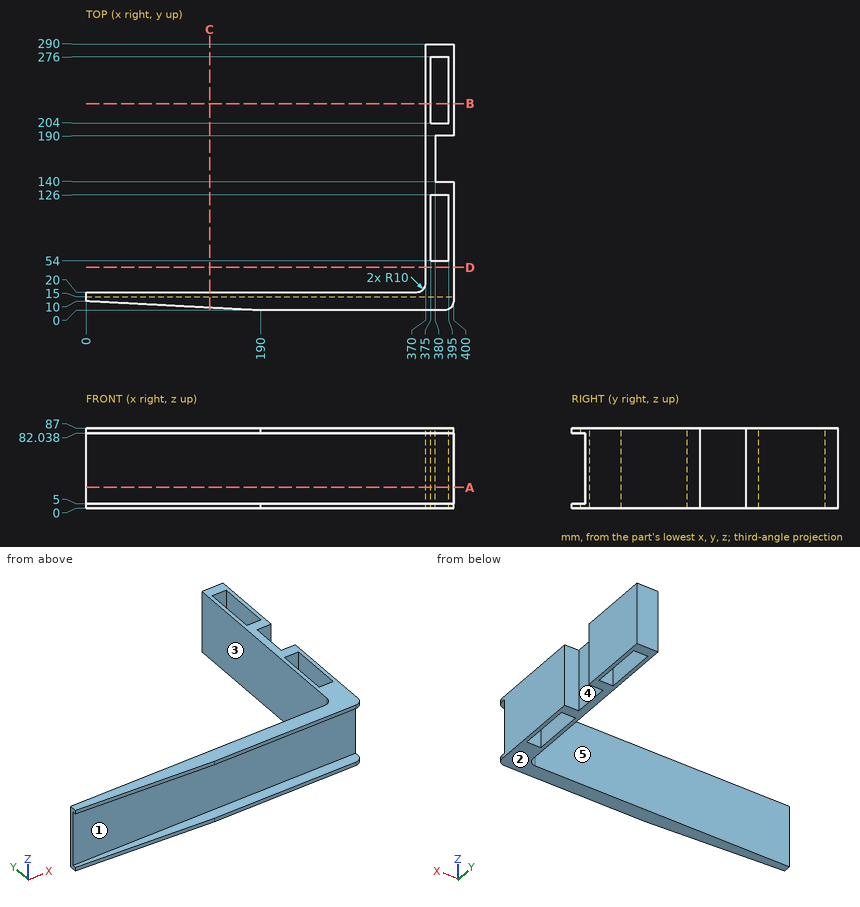
Geometry check sheet. Reference: drawing and pictorial views, mm from the part's lowest x, y, z. A direction names the side the tool comes from. Coordinates: 2 decimals unless noted, no trailing zeros. Order: outer loops, then holes, each group sorted by start corner. A loop starts at its lowest first (then second) coordinate and runs counter-clockwise, first axis right, second up. Notation, with made-up numbers: (71.5, -34.5) -> (93.5, -34.5) arc R35 cw to (93.5, 1.5) -> close; hole circle Ø1 at (-26.75, 48.25). An arc over 180 degrees is marked (long way). Put each result on its own line as item: value. Start each with the question number.
1) Cross-section at B-B (y = 225). Enter the section's corners in (x, z), plus the area to 3 significant figures.
2) Cross-section at A-A (z = 23). Enter the section's corners in (x, y), plus the area to 3 significant figures.
3) Cross-section at D-D (y = 47). Enter the section's corners in (x, z), plus the area to 3 significant figures.
4) Material ranges on L1, parallel to Y at x = 379, z = 29; L2, parallel to X at y = 238.5, z = 41; L3, parallel to Y at x = 158, z = 73, recorded low to high.
5) Go/stop test with flat-tipped pins: pin 1 (1 mm diameter, centred on x = 284, z = 66, fed in from +Y); pin 2 (1.5 mm diameter, centred on x = 331.5, z = 57.5, fed in from -Y). Record where each tip stops, or that it passes through.
6) Cross-section at C-C (x = 134.5). Enter the section's corners in (y, z), plus the area to 3 significant figures.
7) Release check for a two-part mould opening along Y. For the marked faces 3, 4 and 5 record: pulls with the +Y half, pulls with the -Y half, needs draft (parallel to the pull), parting line crosses it, or undercut.
8) Tool access check on the marked faces 1 and 2. Record the directions out of +Z, -Z, +X, -X, +Y, -Y that give a thin tool (end or side, any length) a straight path to the whole face; none if there is none.
Geometry check:
1. outline: (370, 0) -> (375, 0) -> (375, 87) -> (370, 87) -> close; (395, 0) -> (400, 0) -> (400, 87) -> (395, 87) -> close
1. area: 870 mm^2
2. outline: (0, 15) -> (400, 15) -> (400, 140) -> (380, 140) -> (380, 190) -> (400, 190) -> (400, 290) -> (370, 290) -> (370, 30) arc R10 cw to (360, 20) -> (0, 20) -> close; hole (375, 54) -> (395, 54) -> (395, 126) -> (375, 126) -> close; hole (375, 204) -> (395, 204) -> (395, 276) -> (375, 276) -> close
2. area: 6,240 mm^2
3. outline: (370, 0) -> (400, 0) -> (400, 87) -> (370, 87) -> close
3. area: 2,610 mm^2
4. L1: y = 15 to 54, 126 to 204, 276 to 290
4. L2: x = 370 to 375, 395 to 400
4. L3: y = 15 to 20
5. pin 1: stops at y = 20
5. pin 2: stops at y = 15
6. outline: (2.92, 0) -> (20, 0) -> (20, 87) -> (2.92, 87) -> (2.92, 82.04) -> (15, 82.04) -> (15, 5) -> (2.92, 5) -> close
6. area: 555 mm^2
7. face 3: needs draft
7. face 4: undercut
7. face 5: pulls with the +Y half
8. face 1: +X, -X, -Y
8. face 2: -Z, +X, -X, +Y, -Y
